The listing builds one solid part. Answer for the finished solid, in the listing's coordinates (mm). A direction names the side the tool comes from. Give positions to 0.01 mm unless a question says otherwise; leave off trailing zeros. Write each loop counter-clockwise with the first axis right and the second up, starting at its lowest first coordinate (ties: lowest second). Pieces come first, ordered by that corner, then holes. Notation, with made-up numbers: (30, -32) -> (56, -32) arc R15 ccw to (56, -8) -> close; hole circle Ø4 at (51, -33). An arc over 180 degrees is marked (long way). Use CSV: the item, a comma, the result in double quotes. Start each with the question number.
from build123d import *

# Parameters (mm, degrees)
SKETCH_3_R          = 11
EXTRUDE_2_DEPTH     = 35
SKETCH_4_R          = 4
CUT_EXTRUDE_1_DEPTH = 35
SKETCH_5_R          = 2
CUT_EXTRUDE_2_DEPTH = 35


with BuildPart() as part:
    # 草图3 → 凸台-拉伸2 (new body)
    with BuildSketch(Plane.XY):
        Circle(SKETCH_3_R)
    extrude(amount=EXTRUDE_2_DEPTH)

    # 草图4 → 切除-拉伸1 (cut)
    with BuildSketch(Plane.XY.offset(35)):
        Circle(SKETCH_4_R)
    extrude(amount=-CUT_EXTRUDE_1_DEPTH, mode=Mode.SUBTRACT)

    # 草图5 → 切除-拉伸2 (cut)
    with BuildSketch(Plane(origin=(0, 0, 0), x_dir=(1, 0, 0), z_dir=(0, 1, 0))):
        with Locations(Location((0, -6.763631076, 0), (0, 0, 270))):
            Circle(SKETCH_5_R)
        with Locations(Location((0, -28.03443095, 0), (0, 0, 270))):
            Circle(SKETCH_5_R)
    extrude(amount=-CUT_EXTRUDE_2_DEPTH, mode=Mode.SUBTRACT)


solid = part.part
Q1. Flat-ended cylindrical pins translate along their axes: pin 1 Ø2 at (x, z) = (5, 11) entering from -Y; pin 2 Ø4 at (x, z) = (-8.5, 13) entering from -Y; pin 3 Ø4 at (y, z) = (2.5, 22.5) entering from +X. Find the tip coordinate at first contact, or state that the pin passes through.
Q2. Straight lines are drawn through the part: L1, parallel to Z at x = 0, y = -6.25; L2, parallel to Y at x = 0, z = 12.5; L3, parallel to X at y = -0.5, z = 3. For each, find the intervals that lie inside material, in ascending order.
Q3. For faces 4 (the face through (0, -5, 35)), 5 (the face through (0.088, -7.182, 26.036)), determine the directions among +Z, -Z, +X, -X, +Y, -Y from which every point of the face is accessible in a straight line to the end or side of a thin tool.
Q4. Section A-A on x = 0 is taken. Give the vertices of the cut face in (y, z).
Q5. Section D-D on z = 22.5 is taken. Give the vertices of the cut face in (x, y), then the cut area to 3 significant figures.
Q6. The mould has two halves that part along Y. Classify faces 1 (the face through (-0.521, 3.966, 17.745)), 2 (the face through (0.088, -7.182, 4.766)), 3 (the face through (-2.38, -10.74, 17.26)): +Y half, -Y half, draft (parallel to the pull), parting line (faces both ways), or undercut.
Q7. Section C-C on x = 3 is taken. Give the vertices of the cut face in (y, z), then the cut area to 3 significant figures.
Q8. Section B-B on y = 0 is taken. Give the vertices of the cut face in (x, z), then the cut area to 3 significant figures.
Output:
1,pin 1,"y = -10.25"
1,pin 2,"y = -8.87"
1,pin 3,"x = 10.99"
2,L1,"0 to 4.76, 8.76 to 26.03, 30.03 to 35"
2,L2,"-11 to -4, 4 to 11"
2,L3,"-10.99 to -3.97, 3.97 to 10.99"
3,face 4,"+Z, +X, -X, +Y, -Y"
3,face 5,"-Y"
4,outline,"(-11, 0) -> (-4, 0) -> (-4, 4.76) -> (-11, 4.76) -> close; (-11, 8.76) -> (-4, 8.76) -> (-4, 26.03) -> (-11, 26.03) -> close; (-11, 30.03) -> (-4, 30.03) -> (-4, 35) -> (-11, 35) -> close; (4, 0) -> (11, 0) -> (11, 35) -> (4, 35) -> close"
5,outline,"circle Ø22 at (0, 0); hole circle Ø8 at (0, 0)"
5,area,"330 mm²"
6,face 1,"undercut"
6,face 2,"draft"
6,face 3,"parting line"
7,outline,"(-10.58, 0) -> (-2.65, 0) -> (-2.65, 35) -> (-10.58, 35) -> close; (2.65, 0) -> (10.58, 0) -> (10.58, 35) -> (2.65, 35) -> close"
7,area,"556 mm²"
8,outline,"(-11, 0) -> (-4, 0) -> (-4, 35) -> (-11, 35) -> close; (4, 0) -> (11, 0) -> (11, 35) -> (4, 35) -> close"
8,area,"490 mm²"
